CAD build for the part. Positions are in the model's coordinates, mm. Face numbers are marked on the shaded views. A direction names the side the tool comes from. Give positions to 0.01 mm unless a question says otherwise; leave off trailing zeros. Write each loop counter-clockwise with the first axis right and the second up, starting at its lowest first coordinate (ties: lowest second). Pieces come first, ordered by that corner, then holes. Notation, with made-up numbers: (11, -14.75) - (43, -14.75) arc R9 cw to (43, -5.75) - close; hole circle Ø9 at (44.5, -21.5). An arc over 180 degrees is marked (long way). Answer as a JSON object with one key per item and string values.
from build123d import *

# Parameters (mm, degrees)
SKETCH1_R           = 30
BOSS_EXTRUDE1_DEPTH = 15
CUT_EXTRUDE1_DEPTH  = 20
CIRPATTERN1_COUNT   = 3


with BuildPart() as part:
    # Sketch1 → Boss-Extrude1 (new body)
    with BuildSketch(Plane(origin=(0, 0, 0), x_dir=(1, 0, 0), z_dir=(0, 1, 0))):
        with Locations(Location((0, 0, 0), (0, 0, 270))):
            Circle(SKETCH1_R)
    extrude(amount=BOSS_EXTRUDE1_DEPTH)

    # Sketch4 → Cut-Extrude1 (cut)
    with BuildSketch(Plane(origin=(0, 15, -30), x_dir=(-1, 0, 0), z_dir=(0, 0, -1))):
        Polygon((-7.5, -10), (-7.5, -5.75), (-6.65, -5.75), (-6.65, -4.25), (-7.5, -4.25), (-7.5, 0), (7.5, 0), (7.5, -4.25), (6.65, -4.25), (6.65, -5.75), (7.5, -5.75), (7.5, -10), align=None)
    cut_extrude1 = extrude(amount=-CUT_EXTRUDE1_DEPTH, mode=Mode.SUBTRACT)

    # CirPattern1: Cut-Extrude1 ×3 about axis
    cirpattern1_axis = Axis((0, 0, 0), (0, 1, 0))
    for i in range(1, CIRPATTERN1_COUNT):
        add(cut_extrude1.rotate(cirpattern1_axis, i * 360 / CIRPATTERN1_COUNT), mode=Mode.SUBTRACT)


solid = part.part
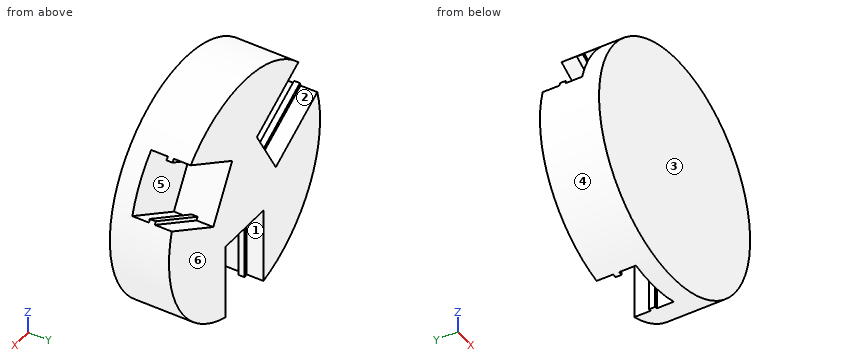
(1) Probe L1, parallel to Y at x = -7, z = -17; L2, parallel to X at y = 6.25, z = 3; L3, parallel to Y at x = 7, z = 8.5. List the from-to ranges inside material, lowest first. Write a range as [from, to].
Answer key:
{"L1": "y = [0, 5], [9.25, 10.75]", "L2": "x = [-29.85, -20.2], [-9.81, 9.81], [20.2, 29.85]", "L3": "y = [0, 5]"}
(2) Saw through at A-A, the plane y = 10. Give the cut face in (x, z), and give its area (3 significant figures).
Answer key:
{"outline": "(-28.66, 8.87) arc R30 ccw to (-6.65, -29.25) - (-6.65, -10) - (6.65, -10) - (6.65, -29.25) arc R30 ccw to (28.66, 8.87) - (11.99, -0.76) - (5.34, 10.76) - (22.01, 20.39) arc R30 ccw to (-22.01, 20.39) - (-5.34, 10.76) - (-11.99, -0.76) - close", "area": "2,040 mm²"}
(3) Saw through at D-D, the plane z = -26. Give the cut face in (x, y), and give its area (3 significant figures).
Answer key:
{"outline": "(-14.97, 0) - (14.97, 0) - (14.97, 15) - (7.5, 15) - (7.5, 10.75) - (6.65, 10.75) - (6.65, 9.25) - (7.5, 9.25) - (7.5, 5) - (-7.5, 5) - (-7.5, 9.25) - (-6.65, 9.25) - (-6.65, 10.75) - (-7.5, 10.75) - (-7.5, 15) - (-14.97, 15) - close", "area": "302 mm²"}
(4) 3-axis set-ups, long thin cutter, end or side, ignore diameter. For the marked faces 1, 2 and 3: which of +Z, -Z, +X, -X, +Y, -Y reach the whole face in a straight line?
Answer key:
{"face 1": "-Z, +Y", "face 2": "+Y", "face 3": "+Z, -Z, +X, -X, -Y"}
(5) Flat gauge pins, fed straight in: P1, Ø3, axis at x = -19, z = 6, coming from the -Y side; P2, Ø4.5, axis at x = -2, z = -19, coming from the +Y side; P3, Ø3, axis at x = -4.5, y = 9.5, coming from the +Z side; P4, Ø3, axis at x = 22, y = 11.5, coming from the -Z side. Where does each tip first touch, or does it go through?
Answer key:
{"P1": "stops at y = 0", "P2": "stops at y = 5", "P3": "stops at z = 29.85", "P4": "stops at z = -21.9"}
(6) Saw through at B-B, the plane x = 0. Give the cut face in (y, z).
Answer key:
{"outline": "(0, -30) - (5, -30) - (5, -10) - (15, -10) - (15, 30) - (0, 30) - close"}
(7) Pull direction X, two halves, no side cores. Call the marked faces 4, 5 and 6: pulls with the +X half, pulls with the -X half, needs draft (parallel to the pull), parting line crosses it, or undercut.
Answer key:
{"face 4": "parting line crosses it", "face 5": "undercut", "face 6": "needs draft"}
(8) Saw through at C-C, the plane z = 13.5. Give the cut face in (x, y), and give its area (3 significant figures).
Answer key:
{"outline": "(-26.79, 0) - (26.79, 0) - (26.79, 5) - (8.38, 5) - (8.38, 9.25) - (10.08, 9.25) - (10.08, 10.75) - (8.38, 10.75) - (8.38, 15) - (-8.38, 15) - (-8.38, 10.75) - (-10.08, 10.75) - (-10.08, 9.25) - (-8.38, 9.25) - (-8.38, 5) - (-26.79, 5) - close", "area": "441 mm²"}
